The model under review builds one solid part; all positions refer to its coordinate system, in mm. A direction names the side the tool comes from. Round coordinates to 2 decimals unless told otherwise and drop trailing zeros. Write each loop counter-clockwise with the first axis right and the second up, starting at its lowest first coordinate (ties: lowest second). Pieces come first, ordered by that corner, then holes. Notation, with made-up numbers: (39, 2.25) -> (72, 2.25) arc R33 ccw to (72, 34.25) -> close; hole circle Ø5 at (-6, -35.5). An arc over 180 degrees is marked (long way). Use CSV: the item, a comma, the result in double quotes. Start each with the question number.
1) Take a section at D-D, the plane x = -15.5. Give the boundary of the cut face in (y, z) (3 decimals), then the cut area to 3 significant figures.
2) For pin 1 Ø1.6 at (x, y) = (28, 2) entering from +Z; pin 2 Ø1 at (y, z) = (1, -4) entering from +X, all flat-tipped, find the tip position at first contact; note any pin that passes through.
3) Take a section at C-C, the plane y = 0.7. Give the boundary of the cut face in (x, z) (3 decimals), then the cut area to 3 significant figures.
4) Take a section at B-B, the plane x = 0. Give the boundary of the cut face in (y, z) (3 decimals).
5) Mouldability with a two-part tool opening along Z and no side actions: class faces 1 (the face through (28, 2, 0)), 2 (the face through (-25, 2, 49)), 3 (the face through (13.8, 2, -3)) as released by +Z, released by -Z, zero draft, split by the parting line, or undercut.
6) Machinability: for faces 4 (the face through (-15.46, 1.61, 3.75)), 5 (the face through (0, 2, -42.375)), which of the approach directions +Z, -Z, +X, -X, +Y, -Y give a long, thin tool a straight path to every point of the face, cutting with its end or side? Answer none if there is none.
7) Take a section at A-A, the plane z = 12.55. Give the boundary of the cut face in (x, y) (3 decimals).
8) Wall thickness on probe 1 along Z at (x, y) = (16.5, 0.25) (3 decimals); probe 2 along X at (y, z) = (0.8, 12.55); probe 3 along X at (y, z) = (1, 101): over which ranges is each line inside the solid? List them lowest first. Write a range as [from, to].
from build123d import *

# Parameters (mm, degrees)
BOSS_EXTRUDE1_DEPTH  = 3.175
SKETCH2_R            = 5
CUT_EXTRUDE1_DEPTH   = 146.820244651
M3_CLEARANCE_HOLE1_D = 3.4
CUT_EXTRUDE2_DEPTH   = 146.820244651


with BuildPart() as part:
    # Sketch1 → Boss-Extrude1 (new body)
    with BuildSketch(Plane(origin=(0, 0, 0), x_dir=(1, 0, 0), z_dir=(0, 1, 0))):
        Polygon((-25, 0), (-25, 42.375), (25, 42.375), (25, 0), (31.35, 0), (31.35, -100), (25, -100), (25, -142.375), (-25, -142.375), (-25, -100), align=None)
    extrude(amount=BOSS_EXTRUDE1_DEPTH)

    # Sketch2 → Cut-Extrude1 (cut, through all)
    with BuildSketch(Plane(origin=(0, 3.175, 0), x_dir=(1, 0, 0), z_dir=(0, 1, 0))):
        with Locations(Location((0, -12.55, 0), (0, 0, 270))):
            Circle(SKETCH2_R)
    extrude(amount=-CUT_EXTRUDE1_DEPTH, mode=Mode.SUBTRACT)

    # M3 Clearance Hole1 (through all)
    with Locations(Plane(origin=(0, 3.175, 0), x_dir=(1, 0, 0), z_dir=(0, 1, 0))):
        with Locations((-15.5, 2.95), (15.5, 2.95), (15.5, -28.05), (-15.5, -28.05)):
            Hole(M3_CLEARANCE_HOLE1_D / 2)

    # Sketch7 → Cut-Extrude2 (cut, through all)
    with BuildSketch(Plane(origin=(0, 3.175, 0), x_dir=(1, 0, 0), z_dir=(0, 1, 0))):
        with BuildLine():
            Line((17.2, 7.95), (17.2, -2.05))
            ThreePointArc((17.2, -2.05), (15.5, -3.75), (13.8, -2.05))
            Line((13.8, -2.05), (13.8, 7.95))
            ThreePointArc((13.8, 7.95), (15.5, 9.65), (17.2, 7.95))
        make_face()
        with BuildLine():
            Line((-13.8, 7.95), (-13.8, -2.05))
            ThreePointArc((-13.8, -2.05), (-15.5, -3.75), (-17.2, -2.05))
            Line((-17.2, -2.05), (-17.2, 7.95))
            ThreePointArc((-17.2, 7.95), (-15.5, 9.65), (-13.8, 7.95))
        make_face()
        with BuildLine():
            Line((17.2, -33.05), (17.2, -23.05))
            ThreePointArc((17.2, -23.05), (15.5, -21.35), (13.8, -23.05))
            Line((13.8, -23.05), (13.8, -33.05))
            ThreePointArc((13.8, -33.05), (15.5, -34.75), (17.2, -33.05))
        make_face()
        with BuildLine():
            Line((-13.8, -33.05), (-13.8, -23.05))
            ThreePointArc((-13.8, -23.05), (-15.5, -21.35), (-17.2, -23.05))
            Line((-17.2, -23.05), (-17.2, -33.05))
            ThreePointArc((-17.2, -33.05), (-15.5, -34.75), (-13.8, -33.05))
        make_face()
    extrude(amount=-CUT_EXTRUDE2_DEPTH, mode=Mode.SUBTRACT)


solid = part.part
Values found:
1,outline,"(0, -42.375) -> (3.175, -42.375) -> (3.175, -9.65) -> (0, -9.65) -> close; (0, 3.75) -> (3.175, 3.75) -> (3.175, 21.35) -> (0, 21.35) -> close; (0, 34.75) -> (3.175, 34.75) -> (3.175, 142.375) -> (0, 142.375) -> close"
1,area,"501 mm²"
2,pin 1,"z = 100"
2,pin 2,"x = 25"
3,outline,"(-25, -42.375) -> (25, -42.375) -> (25, 0) -> (31.35, 0) -> (31.35, 100) -> (25, 100) -> (25, 142.375) -> (-25, 142.375) -> close; hole (-17.2, -7.95) arc R1.7 ccw to (-13.8, -7.95) -> (-13.8, 2.05) arc R1.7 ccw to (-17.2, 2.05) -> close; hole (-17.2, 23.05) arc R1.7 ccw to (-13.8, 23.05) -> (-13.8, 33.05) arc R1.7 ccw to (-17.2, 33.05) -> close; hole circle Ø10 at (0, 12.55); hole (13.8, -7.95) arc R1.7 ccw to (17.2, -7.95) -> (17.2, 2.05) arc R1.7 ccw to (13.8, 2.05) -> close; hole (13.8, 23.05) arc R1.7 ccw to (17.2, 23.05) -> (17.2, 33.05) arc R1.7 ccw to (13.8, 33.05) -> close"
3,area,"9,620 mm²"
4,outline,"(0, -42.375) -> (3.175, -42.375) -> (3.175, 7.55) -> (0, 7.55) -> close; (0, 17.55) -> (3.175, 17.55) -> (3.175, 142.375) -> (0, 142.375) -> close"
5,face 1,"released by -Z"
5,face 2,"zero draft"
5,face 3,"undercut"
6,face 4,"+Y, -Y"
6,face 5,"-Z, +X, -X, +Y, -Y"
7,outline,"(-25, 0) -> (-5, 0) -> (-5, 3.175) -> (-25, 3.175) -> close; (5, 0) -> (31.35, 0) -> (31.35, 3.175) -> (5, 3.175) -> close"
8,probe 1,"[-42.375, -9.325], [3.425, 21.675], [34.425, 142.375]"
8,probe 2,"[-25, -5], [5, 31.35]"
8,probe 3,"[-25, 25]"
